Source: CAD feature listing. Evaluate the final solid. Frame: model axes, mm. A direction names the side the tool comes from. Give positions to 0.01 mm unless a question says otherwise; leave off trailing zeros. Loops run counter-clockwise (first coordinate to the right, second up) from the corner with the lowest first, then second, coordinate; pieces in that order, holes last.
from build123d import *

# Parameters (mm, degrees)
PAD_DEPTH       = 6
SKETCH001_R     = 20.3
POCKET_DEPTH    = 4
POCKET001_DEPTH = 4
POCKET002_DEPTH = 3
SKETCH004_R     = 1.5
POCKET003_DEPTH = 6.001
SKETCH005_R     = 10
SKETCH005_R_2   = 3.6
PAD001_DEPTH    = 4
FILLET_R        = 1
CHAMFER_SIZE    = 1


with BuildPart() as part:
    # Sketch → Pad (new body)
    with BuildSketch(Plane.XY):
        with BuildLine():
            Line((-30, 27), (-30, -27))
            ThreePointArc((-30, -27), (-29.12132, -29.12132), (-27, -30))
            Line((-27, -30), (27, -30))
            ThreePointArc((27, -30), (29.12132, -29.12132), (30, -27))
            Line((30, -27), (30, 27))
            ThreePointArc((30, 27), (29.12132, 29.12132), (27, 30))
            Line((27, 30), (-27, 30))
            ThreePointArc((-27, 30), (-29.12132, 29.12132), (-30, 27))
        make_face()
    extrude(amount=PAD_DEPTH)

    # Sketch001 (on Face10 of Pad) → Pocket (cut)
    with BuildSketch(Plane.XY.offset(6)):
        Circle(SKETCH001_R)
    extrude(amount=-POCKET_DEPTH, mode=Mode.SUBTRACT)

    # Sketch002 (on Face5 of Pocket) → Pocket001 (cut)
    with BuildSketch(Plane.XY.offset(6)):
        Polygon((-22.5, 1.5), (-1.5, 1.5), (-1.5, 22.5), (1.5, 22.5), (1.5, 1.5), (22.5, 1.5), (22.5, -1.5), (1.5, -1.5), (1.5, -22.5), (-1.5, -22.5), (-1.5, -1.5), (-22.5, -1.5), align=None)
    extrude(amount=-POCKET001_DEPTH, mode=Mode.SUBTRACT)

    # Sketch003 (on Face5 of Pocket001) → Pocket002 (cut)
    with BuildSketch(Plane.XY.offset(6)):
        with BuildLine():
            Line((-30, 27), (-30, -27))
            ThreePointArc((-30, -27), (-29.12132, -29.12132), (-27, -30))
            Line((-27, -30), (27, -30))
            ThreePointArc((27, -30), (29.12132, -29.12132), (30, -27))
            Line((30, -27), (30, 27))
            ThreePointArc((30, 27), (29.12132, 29.12132), (27, 30))
            Line((27, 30), (-27, 30))
            ThreePointArc((-27, 30), (-29.12132, 29.12132), (-30, 27))
        make_face()
        with BuildLine():
            Line((-27, 24), (-27, -24))
            ThreePointArc((-27, -24), (-26.12132, -26.12132), (-24, -27))
            Line((-24, -27), (24, -27))
            ThreePointArc((24, -27), (26.12132, -26.12132), (27, -24))
            Line((27, -24), (27, 24))
            ThreePointArc((27, 24), (26.12132, 26.12132), (24, 27))
            Line((24, 27), (-24, 27))
            ThreePointArc((-24, 27), (-26.12132, 26.12132), (-27, 24))
        make_face(mode=Mode.SUBTRACT)
    extrude(amount=-POCKET002_DEPTH, mode=Mode.SUBTRACT)

    # Sketch004 (on Face19 of Pocket002) → Pocket003 (cut, through all)
    with BuildSketch(Plane.XY.offset(6)):
        with Locations((-23, 23)):
            Circle(SKETCH004_R)
        with Locations((-23, -23)):
            Circle(SKETCH004_R)
        with Locations((23, -23)):
            Circle(SKETCH004_R)
        with Locations((23, 23)):
            Circle(SKETCH004_R)
    extrude(amount=-POCKET003_DEPTH, mode=Mode.SUBTRACT)

    # Sketch005 (on Face40 of Pocket003) → Pad001 (join)
    with BuildSketch(Plane.XY.offset(2)):
        Circle(SKETCH005_R)
        Circle(SKETCH005_R_2, mode=Mode.SUBTRACT)
    extrude(amount=PAD001_DEPTH)

    # Fillet
    fillet_edges = [part.edges().sort_by_distance(p)[0] for p in [
        (-10, 0, 6),
    ]]
    fillet(fillet_edges, radius=FILLET_R)

    # Chamfer
    chamfer_edges = [part.edges().sort_by_distance(p)[0] for p in [
        (-3.6, 0, 6),
    ]]
    chamfer(chamfer_edges, length=CHAMFER_SIZE)


solid = part.part
1) Cut plane A-A (z = 3.9). State how many separate pieces and enclosed holes the cut face has, and give its area (3 significant figures).
Checks:
separate pieces: 2
enclosed holes: 6
area: 1,830 mm2
2) Cut plane C-C (y = -19.5). Return loops of the section in (x, z), and give its area (3 significant figures).
Checks:
outline: (-30, 0) - (30, 0) - (30, 3) - (27, 3) - (27, 6) - (5.64, 6) - (5.64, 2) - (-5.64, 2) - (-5.64, 6) - (-27, 6) - (-27, 3) - (-30, 3) - close
area: 297 mm2
3) Reachability of faces 1 (the cylindrical face through (-14.211, 14.497, 4.028)), 2 (the cylindrical face through (-26.14, -26.1, 4.52)), 3 (the cylindrical face through (26.1, -26.14, 4.52)), 4 (the cylindrical face through (-26.1, 26.14, 4.52)), 5 (the flat face through (0, 27, 5)) from +Z, -Z, +X, -X, +Y, -Y: full face, straight path, thin tool, end or side. Return the list, or none.
Checks:
face 1: +Z
face 2: +Z, -X, -Y
face 3: +Z, +X, -Y
face 4: +Z, -X, +Y
face 5: +Z, +X, -X, +Y
4) Pull-direction query (X, two-part tool) for faces 6 (the flat face through (30, 0, 1)), 7 (the flat face through (0, -27, 5)), 8 (the cylindrical face through (14.211, -14.497, 4.028)), 9 (the flat face through (-30, 0, 1)); classes: released by +X, released by -X, zero draft, split by the parting line, or undercut.
Checks:
face 6: released by +X
face 7: zero draft
face 8: undercut
face 9: released by -X
5) Cut plane D-D (x = 0). Return loops of the section in (y, z), and give its area (3 significant figures).
Checks:
outline: (-30, 0) - (30, 0) - (30, 3) - (27, 3) - (27, 6) - (22.5, 6) - (22.5, 2) - (10, 2) - (10, 5) arc R1 ccw to (9, 6) - (4.6, 6) - (3.6, 5) - (3.6, 2) - (-3.6, 2) - (-3.6, 5) - (-4.6, 6) - (-9, 6) arc R1 ccw to (-10, 5) - (-10, 2) - (-22.5, 2) - (-22.5, 6) - (-27, 6) - (-27, 3) - (-30, 3) - close
area: 212 mm2
6) Ray query, probe 1 along Y at (x, z) = (-23, 1.3); probe 2 along Y at (x, z) = (23, 4.2); probe 3 along Y at (x, z) = (0, 3.5). Return the intervals inside material, ascending.
Checks:
probe 1: y = -30 to -24.5, -21.5 to 21.5, 24.5 to 30
probe 2: y = -27 to -24.5, -21.5 to 21.5, 24.5 to 27
probe 3: y = -27 to -22.5, -10 to -3.6, 3.6 to 10, 22.5 to 27
7) Cut plane B-B (x = 14). Return loops of the section in (y, z).
Checks:
outline: (-30, 0) - (30, 0) - (30, 3) - (27, 3) - (27, 6) - (14.7, 6) - (14.7, 2) - (-14.7, 2) - (-14.7, 6) - (-27, 6) - (-27, 3) - (-30, 3) - close
8) Contact query for flat-ended pins moving along their axis: P1, Ø2, axis at x = -1.5, y = 1, coming from the +Z side; P2, Ø1.5, axis at x = 8, z = 4.5, coming from the -Y side; P3, Ø1.1, axis at y = 21, z = 4, coming from the -X side. Output: stop coordinate, or through.
Checks:
P1: stops at z = 2
P2: stops at y = -27
P3: stops at x = -27
